from build123d import *

# Parameters (mm, degrees)
SALIENTE_EXTRUIR1_DEPTH = 8
REDONDEO1_R             = 1
CROQUIS2_R              = 1.5
CORTAR_EXTRUIR1_DEPTH   = 35.871191617
CROQUIS3_R              = 10.95
CORTAR_EXTRUIR2_DEPTH   = 6
CROQUIS4_R              = 4.25
CROQUIS4_R_2            = 1.775
CORTAR_EXTRUIR3_DEPTH   = 29.913664638


with BuildPart() as part:
    # Croquis1 → Saliente-Extruir1 (new body)
    with BuildSketch(Plane.XY):
        with BuildLine():
            Line((0, 14), (24, 14))
            Line((24, 14), (24, 10))
            Line((24, 10), (9.797958971, 10))
            ThreePointArc((9.797958971, 10), (0, -14), (-9.797958971, 10))
            Line((-9.797958971, 10), (-24, 10))
            Line((-24, 10), (-24, 14))
            Line((-24, 14), (0, 14))
        make_face()
    extrude(amount=SALIENTE_EXTRUIR1_DEPTH)

    # Redondeo1
    redondeo1_edges = [part.edges().sort_by_distance(p)[0] for p in [
        (-9.797958971, 10, 4),
        (-24, 10, 4),
        (24, 10, 4),
        (9.797958971, 10, 4),
        (-16.898979486, 10, 8),
        (0, -14, 8),
        (-16.898979486, 10, 0),
        (16.898979486, 10, 8),
        (16.898979486, 10, 0),
        (0, -14, 0),
    ]]
    fillet(redondeo1_edges, radius=REDONDEO1_R)

    # Croquis2 → Cortar-Extruir1 (cut, through all)
    with BuildSketch(Plane.XZ.offset(-10)):
        with Locations(Location((-18.949489743, 4, 0), (0, 0, 270))):
            Circle(CROQUIS2_R)
        with Locations(Location((18.949489743, 4, 0), (0, 0, 270))):
            Circle(CROQUIS2_R)
    extrude(amount=-CORTAR_EXTRUIR1_DEPTH, mode=Mode.SUBTRACT)

    # Croquis3 → Cortar-Extruir2 (cut)
    with BuildSketch(Plane.XY.offset(8)):
        Circle(CROQUIS3_R)
    extrude(amount=-CORTAR_EXTRUIR2_DEPTH, mode=Mode.SUBTRACT)

    # Croquis4 → Cortar-Extruir3 (cut, through all)
    with BuildSketch(Plane(origin=(0, 0, 0), x_dir=(-1, 0, 0), z_dir=(0, 0, -1))):
        Circle(CROQUIS4_R)
        with Locations((7.5, 0)):
            Circle(CROQUIS4_R_2)
        with Locations((-7.5, 0)):
            Circle(CROQUIS4_R_2)
    extrude(amount=-CORTAR_EXTRUIR3_DEPTH, mode=Mode.SUBTRACT)


solid = part.part
The model under review builds one solid part; all positions refer to its coordinate system, in mm. A direction names the side the tool comes from. Give positions to 0.01 mm unless a question says otherwise; leave off trailing zeros. Loops run counter-clockwise (first coordinate to the right, second up) from the corner with the lowest first, then second, coordinate; pieces in that order, holes last. Notation, with made-up numbers: (-10, -18) -> (20, -18) arc R17 cw to (20, 2) -> close; hole circle Ø11 at (-14, 76.25). An arc over 180 degrees is marked (long way). Write each question's results on one line, items separated by ' | '.
1) Take a section at B-B, the plane z = 4. Give the boundary of the cut face in (x, y), plus the area to 3 significant figures.
Conclusion:
outline: (-24, 11) arc R1 ccw to (-23, 10) -> (-20.45, 10) -> (-20.45, 14) -> (-24, 14) -> close; (-17.45, 10) -> (-12, 10) arc R1 cw to (-11.2, 8.4) arc R14 ccw (long way) to (11.2, 8.4) arc R1 cw to (12, 10) -> (17.45, 10) -> (17.45, 14) -> (-17.45, 14) -> close; (20.45, 10) -> (23, 10) arc R1 ccw to (24, 11) -> (24, 14) -> (20.45, 14) -> close; hole circle Ø21.9 at (0, 0) | area: 355 mm^2
2) Take a section at D-D, the plane x = 21.5. Give the boundary of the cut face in (y, z), plus the area to 3 significant figures.
Conclusion:
outline: (10, 1) arc R1 ccw to (11, 0) -> (14, 0) -> (14, 8) -> (11, 8) arc R1 ccw to (10, 7) -> close | area: 31.6 mm^2
3) For line 1 along X through (y, z) = (11.9, 4); line 2 along Y through (x, z) = (0, 0.9); line 3 along Y through (x, z) = (0, 3.8), list the stretches that pass through material, from the lowest coordinate up. Write a range as from..to.
Conclusion:
line 1: x = -24..-20.45, -17.45..17.45, 20.45..24 | line 2: y = -13.99..-4.25, 4.25..14 | line 3: y = -14..-10.95, 10.95..14
4) Take a section at A-A, the plane x = 0. Give the boundary of the cut face in (y, z).
Conclusion:
outline: (-14, 1) arc R1 ccw to (-13, 0) -> (-4.25, 0) -> (-4.25, 2) -> (-10.95, 2) -> (-10.95, 8) -> (-13, 8) arc R1 ccw to (-14, 7) -> close; (4.25, 0) -> (14, 0) -> (14, 8) -> (10.95, 8) -> (10.95, 2) -> (4.25, 2) -> close
5) Tool access review of faces 4 (the face through (17.916, 10.285, 7.699)), 5 (the face through (17.916, 10.285, 0.301)), 6 (the face through (-8.69, -6.66, 5.04)), 7 (the face through (0, 12, 8)): name each direction out of +Z, -Z, +X, -X, +Y, -Y from which nothing blocks a thin tool from reaching the whole face with its end or side.
Conclusion:
face 4: +Z, +X | face 5: -Z, +X | face 6: +Z | face 7: +Z, +X, -X, +Y, -Y
6) Insertion check: pin 1 Ø4 at (y, z) = (1, 2) entering from +X; pin 2 Ø1.8 at (x, z) = (18, 4) entering from -Y; pin 3 Ø2 at (y, z) = (-8.5, 1) entering from -X. Each pin has a flat end and moves straight along its axis. Give the tip position at first contact, or say it passes through.
Conclusion:
pin 1: stops at x = 14 | pin 2: stops at y = 10 | pin 3: stops at x = -11.82
7) Take a section at C-C, the plane y = 0. Count the separate pieces of the cut face and the enclosed holes in it, plus the area to 3 significant figures.
Conclusion:
separate pieces: 4 | enclosed holes: 0 | area: 60.5 mm^2
8) Draft analysis for pull direction Y (two halves, no side actions). For faces 1 (the face through (0, -14, 4)), 2 (the face through (24, 13, 4)), 3 (the face through (23.715, 10.301, 4.056)), state which applies: pulls with the +Y half, pulls with the -Y half, needs draft (parallel to the pull), parting line crosses it, or undercut.
Conclusion:
face 1: undercut | face 2: needs draft | face 3: pulls with the -Y half
